Source: three-view drawing plus pictorial views. Frame: mm from the lowest corner of the part. Give positions to 0.01 mm unless a question says otherwise; leave off trailing zeros. Loops run counter-clockwise (first coordinate to the right, second up) from the corner with the lowest first, then second, coordinate; pieces in that order, holes last. Notation, with made-up numbers: (5.5, -2.75) -> (51.5, -2.75) arc R16 cw to (51.5, 28.25) -> close; hole circle Ø8 at (37, -37.75). An arc over 180 degrees is marked (long way). Answer in a Markdown table with one row per item. Add a question column.
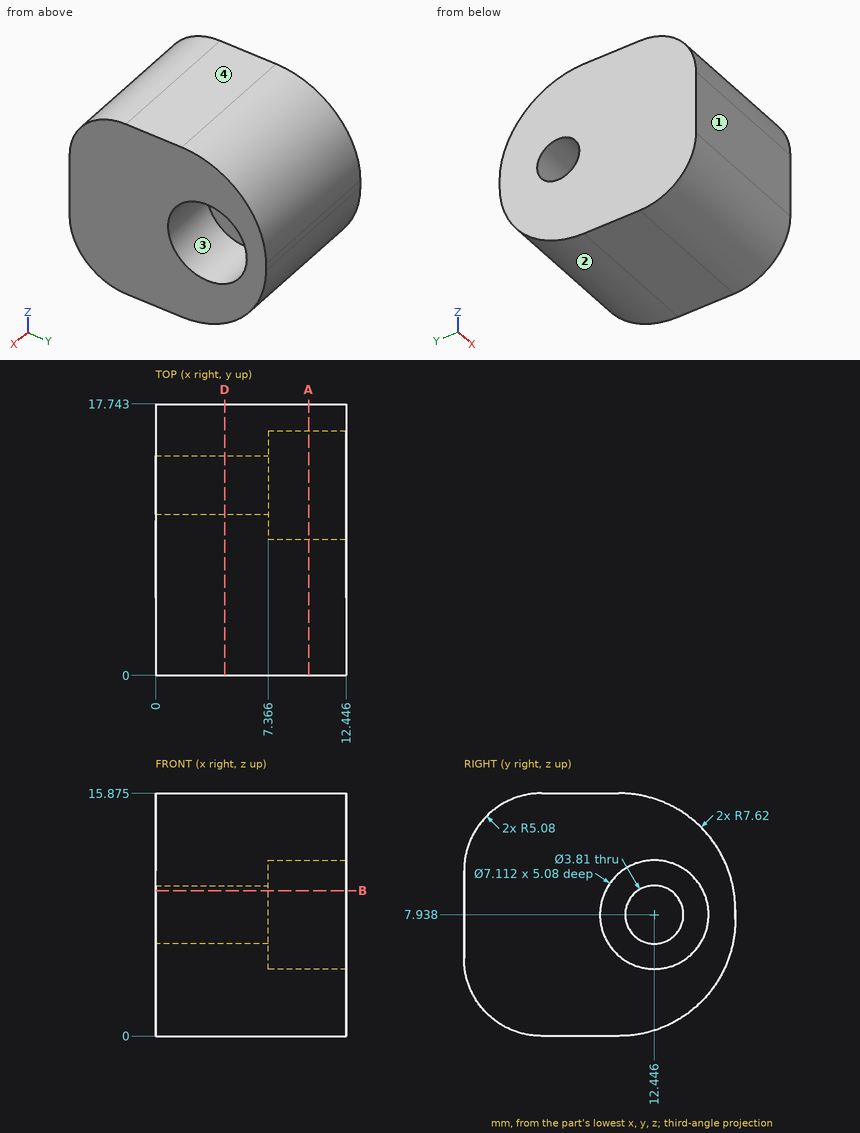
(1) Material intervals for line 1 along Y through (x, z) = (9, 6.5) (1 decimal); line 2 along Z through (x, y) = (2, 11.25) (1 decimal); line 3 along Y through (x, z) = (11, 9) (1 decimal), sorted ascending. Write a range as from..to.
(2) Cut plane B-B on z = 9.5. Return the cut outline in (x, y) (1 decimal), then the cut area to 3 significant figures.
(3) Cut plane A-A on x = 10. Return the cut outline in (y, z) (1 decimal).
(4) Draft query along Z for the marked faces 1, 2, 3 and 4. Return one class per face: +Z half, -Z half, draft (parallel to the pull), parting line (faces both ways), or undercut.
(5) Cut plane D-D on x = 4.5. Return the cut outline in (y, z) (1 decimal).
(6) Pin query (flat end, axial travel): pin 1 Ø2 at (y, z) = (11.5, 9) entering from +X; pin 2 Ø5.5 at (y, z) = (12.45, 7.94) entering from -X. Return the tip coordinate at first contact, or that it passes through.
Answer list:
| question | item | result |
|---|---|---|
| 1 | line 1 | y = 0..9.2, 15.7..17.7 |
| 1 | line 2 | z = 0.1..6.5, 9.4..15.8 |
| 1 | line 3 | y = 0..9.1, 15.8..17.7 |
| 2 | outline | (0, 0) -> (12.4, 0) -> (12.4, 9.3) -> (7.4, 9.3) -> (7.4, 11.4) -> (0, 11.4) -> close; (0, 13.5) -> (7.4, 13.5) -> (7.4, 15.6) -> (12.4, 15.6) -> (12.4, 17.6) -> (0, 17.6) -> close |
| 2 | area | 171 mm² |
| 3 | outline | (0, 5.1) arc R5.1 ccw to (5.1, 0) -> (10.1, 0) arc R7.6 ccw to (17.7, 7.6) -> (17.7, 8.3) arc R7.6 ccw to (10.1, 15.9) -> (5.1, 15.9) arc R5.1 ccw to (0, 10.8) -> close; hole circle Ø7.1 at (12.4, 7.9) |
| 4 | face 1 | draft |
| 4 | face 2 | -Z half |
| 4 | face 3 | undercut |
| 4 | face 4 | +Z half |
| 5 | outline | (0, 5.1) arc R5.1 ccw to (5.1, 0) -> (10.1, 0) arc R7.6 ccw to (17.7, 7.6) -> (17.7, 8.3) arc R7.6 ccw to (10.1, 15.9) -> (5.1, 15.9) arc R5.1 ccw to (0, 10.8) -> close; hole circle Ø3.8 at (12.4, 7.9) |
| 6 | pin 1 | stops at x = 7.37 |
| 6 | pin 2 | stops at x = 0 |
